Source: CAD feature listing. Evaluate the final solid. Frame: model axes, mm. Round coordinates to 2 decimals unless told otherwise and drop trailing zeros. Write each loop counter-clockwise with the first axis right and the second up, starting at its lowest first coordinate (ties: lowest second). Pieces come first, ordered by that corner, then holes.
from build123d import *

# Parameters (mm, degrees)
F0_W     = 1300
F0_H     = 700
F0_W_2   = 1260
F0_H_2   = 660
F1_DEPTH = 20
F2_W     = 40
F2_H     = 20
F3_DEPTH = 6


with BuildPart() as f1:
    # F0 (on Front) → F1 (new body)
    with BuildSketch(Plane.XZ):
        Rectangle(F0_W, F0_H)
        Rectangle(F0_W_2, F0_H_2, mode=Mode.SUBTRACT)
    extrude(amount=F1_DEPTH)

    # F2 (on Front) → F3 (join)
    with BuildSketch(Plane.XZ):
        with Locations((670, -290)):
            Rectangle(F2_W, F2_H)
    extrude(amount=F3_DEPTH)

    # F4: F1 across plane


with BuildPart() as f1_1:
    add(f1.part)
    add(f1.part.mirror(Plane.XY))

    # F5: F1 across plane


with BuildPart() as f1_2:
    add(f1_1.part)
    add(f1_1.part.mirror(Plane.YZ))


solid = f1_2.part
1) Section query C-C on z = -102.5. Return the cut outline in (x, y), then the cut area to 3 significant figures.
Taken from the geometry:
outline: (-650, -20) - (-630, -20) - (-630, 0) - (-650, 0) - close; (630, -20) - (650, -20) - (650, 0) - (630, 0) - close
area: 800 mm2
2) Section query B-B on y = -11.5. Return the cut outline in (x, z), then the cut area to 3 significant figures.
Taken from the geometry:
outline: (-650, -350) - (650, -350) - (650, 350) - (-650, 350) - close; hole (-630, -330) - (630, -330) - (630, 330) - (-630, 330) - close
area: 78,400 mm2
3) Material intervals for line 1 (X direction, y = -9.25, z = -27); line 2 (Z direction, x = -513.5, y = -7.25), sorted ascending.
Taken from the geometry:
line 1: x = -650 to -630, 630 to 650
line 2: z = -350 to -330, 330 to 350
4) Contact query for flat-ended pins moving along their axis: P1, Ø1, axis at y = -7.5, z = -62.5, coming from the +X side; P2, Ø6, axis at x = -673.5, z = -289, coming from the -Y side; P3, Ø5, axis at x = -678.5, y = -3.5, coming from the -Z side. Output: stop coordinate, or through.
Taken from the geometry:
P1: stops at x = 650
P2: stops at y = -6
P3: stops at z = -300
5) Section query A-A on x = 260. Return the cut outline in (y, z).
Taken from the geometry:
outline: (-20, -350) - (0, -350) - (0, -330) - (-20, -330) - close; (-20, 330) - (0, 330) - (0, 350) - (-20, 350) - close
